Geometry: final body of the model. Coordinates: model frame, mm. A direction names the side the tool comes from. Round coordinates to 2 decimals unless told otherwise and drop trailing zeros. Write each loop counter-clockwise with the first axis right and the second up, starting at its lowest first coordinate (ties: lowest second). Pieces come first, ordered by that corner, then holes. Notation, with made-up numbers: M -22,66 L -13,66 A29 cw -13,90 Z; hole C 10.25,71 d4. An arc over 180 degrees is marked long. Put each result on its own line as item: value. Start each with the question number.
```python
from build123d import *

# Parameters (mm, degrees)
F0_W         = 127
F0_H         = 88.9
F1_DEPTH     = 50.8
F3_DEPTH     = 76.2
F4_W         = 76.2
F4_H         = 25.4
F5_DEPTH     = 38.1
F7_DEPTH     = 38.1
F8_T1_DEPTH  = 76.2
F8_T3_DEPTH  = 38.1
F8_T5_DEPTH  = 74.8723933942
F8_T8_ANGLE  = 242.9501193557
F8_T10_ANGLE = 242.9501193557
F8_T15_DEPTH = 38.1
F8_S16_R     = 24.2542650998
F8_T17_DEPTH = 21
F8_T21_DEPTH = 88.9
F8_S22_R     = 24.2542650998
F8_T23_DEPTH = 46
F8_T30_DEPTH = 88.9
F8_S32_R     = 29.6655396369
F8_T33_DEPTH = 46
F8_T36_DEPTH = 38.1
F8_S38_R     = 29.6655396369
F8_T39_DEPTH = 21


# Not quite as in the source:
# - a fillet or chamfer that OpenCascade refuses, or shapes differently, is made with other operations: its cross-section is extruded or revolved along the edge and cut away or added


with BuildPart() as f1:
    # F0 (on Top) → F1 (new body)
    with BuildSketch(Plane.XY):
        with Locations((0.947636019, -9.969078747)):
            Rectangle(F0_W, F0_H)
    extrude(amount=F1_DEPTH)

    # F2 (on face) → F3 (cut)
    with BuildSketch(Plane.XY.offset(50.8)):
        with BuildLine():
            Line((21.7591244727, 34.480921253), (-28.0215628445, 34.480921253))
            ThreePointArc((-28.0215628445, 34.480921253), (-3.1312191859, 8.6101276845), (21.7591244727, 34.480921253))
        make_face()
    extrude(amount=-F3_DEPTH, mode=Mode.SUBTRACT)

    # F4 (on face) → F5 (cut)
    with BuildSketch(Plane.XY.offset(50.8)):
        with Locations((0.8347104251, -41.719078747)):
            Rectangle(F4_W, F4_H)
    extrude(amount=-F5_DEPTH, mode=Mode.SUBTRACT)

    # F6 (on face) → F7 (cut)
    with BuildSketch(Plane.XY.offset(50.8)):
        with BuildLine():
            Line((-62.552363981, -54.419078747), (-49.9088267779, -54.419078747))
            Line((-49.9088267779, -54.419078747), (-49.9088267779, -29.019078747))
            ThreePointArc((-49.9088267779, -29.019078747), (-39.401677619, -18.2031822516), (-35.5692207813, -3.619078747))
            Line((-35.5692207813, -3.619078747), (-35.5692207813, 34.480921253))
            Line((-35.5692207813, 34.480921253), (-62.552363981, 34.480921253))
            Line((-62.552363981, 34.480921253), (-62.552363981, -54.419078747))
        make_face()
        with BuildLine():
            Line((51.6911732221, -27.8206840158), (51.6911732221, -54.419078747))
            Line((51.6911732221, -54.419078747), (64.447636019, -54.419078747))
            Line((64.447636019, -54.419078747), (64.447636019, 34.480921253))
            Line((64.447636019, 34.480921253), (29.0343053639, 34.480921253))
            Line((29.0343053639, 34.480921253), (29.0343053639, -3.619078747))
            ThreePointArc((29.0343053639, -3.619078747), (35.5824546884, -20.1950505038), (51.6911732221, -27.8206840158))
        make_face()
    extrude(amount=-F7_DEPTH, mode=Mode.SUBTRACT)

    # F8: fillet of radius 5.08 on 8 edges, made by hand

    # F8_s2 → F8_t1 (cut)
    with BuildSketch(Plane.YZ.offset(-37.2652895749)):
        with BuildLine():
            ThreePointArc((-23.939078747, 50.8), (-27.5311811954, 49.3121024484), (-29.019078747, 45.72))
            Line((-29.019078747, 45.72), (-29.019078747, 50.8))
            Line((-29.019078747, 50.8), (-23.939078747, 50.8))
        make_face()
        with BuildLine():
            ThreePointArc((-54.419078747, 7.62), (-52.9311811954, 11.2121024484), (-49.339078747, 12.7))
            Line((-49.339078747, 12.7), (-54.419078747, 12.7))
            Line((-54.419078747, 12.7), (-54.419078747, 7.62))
        make_face()
    extrude(amount=F8_T1_DEPTH, mode=Mode.SUBTRACT)

    # F8_s4 → F8_t3 (cut)
    with BuildSketch(Plane.XZ.offset(29.019078747)):
        with BuildLine():
            ThreePointArc((-42.3452895749, 50.8), (-38.7531871264, 49.3121024484), (-37.2652895749, 45.72))
            Line((-37.2652895749, 45.72), (-37.2652895749, 50.8))
            Line((-37.2652895749, 50.8), (-42.3452895749, 50.8))
        make_face()
        with BuildLine():
            ThreePointArc((44.0147104251, 50.8), (40.4226079767, 49.3121024484), (38.9347104251, 45.72))
            Line((38.9347104251, 45.72), (38.9347104251, 50.8))
            Line((38.9347104251, 50.8), (44.0147104251, 50.8))
        make_face()
    extrude(amount=F8_T3_DEPTH, mode=Mode.SUBTRACT)

    # F8_s6 → F8_t5 (cut)
    with BuildSketch(Plane.XY.offset(-12.0361966971)):
        with BuildLine():
            ThreePointArc((26.5736031516, 34.480921253), (23.2372411895, 33.2317291127), (21.5417284952, 30.0985152915))
            ThreePointArc((21.5417284952, 30.0985152915), (21.7471113974, 32.2849220687), (21.7591244727, 34.480921253))
            Line((21.7591244727, 34.480921253), (26.5736031516, 34.480921253))
        make_face()
        with BuildLine():
            ThreePointArc((-32.8360415234, 34.480921253), (-29.4996795612, 33.2317291127), (-27.804166867, 30.0985152915))
            ThreePointArc((-27.804166867, 30.0985152915), (-28.0095497691, 32.2849220687), (-28.0215628445, 34.480921253))
            Line((-28.0215628445, 34.480921253), (-32.8360415234, 34.480921253))
        make_face()
    extrude(amount=F8_T5_DEPTH, mode=Mode.SUBTRACT)

    # F8_s7 → F8_t8 (revolve, cut)
    with BuildSketch(Plane(origin=(14.0725928873, 22.9868383553, 0), x_dir=(0, 0, 1), z_dir=(0.5221273689, 0.8528675224, 0))):
        with BuildLine():
            ThreePointArc((45.72, -45.0806506369), (49.3121024484, -46.5685481884), (50.8, -50.1606506369))
            Line((50.8, -50.1606506369), (50.8, -45.0806506369))
            Line((50.8, -45.0806506369), (45.72, -45.0806506369))
        make_face()
    revolve(axis=Axis((-3.1312191859, 33.5190498615, 50.8), (0, 0, 1)), revolution_arc=F8_T8_ANGLE, mode=Mode.SUBTRACT)

    # F8_s9 → F8_t10 (revolve, cut)
    with BuildSketch(Plane(origin=(14.0725928873, 22.9868383553, 0), x_dir=(0, 0, 1), z_dir=(0.5221273689, 0.8528675224, 0))):
        with BuildLine():
            ThreePointArc((0, -50.1606506369), (1.4878975516, -46.5685481884), (5.08, -45.0806506369))
            Line((5.08, -45.0806506369), (0, -45.0806506369))
            Line((0, -45.0806506369), (0, -50.1606506369))
        make_face()
    revolve(axis=Axis((-3.1312191859, 33.5190498615, 0), (0, 0, 1)), revolution_arc=F8_T10_ANGLE, mode=Mode.SUBTRACT)


with BuildPart() as f8_tool13:
    # F8_s14 → F8_t15 (new body)
    with BuildSketch(Plane.XZ.offset(54.419078747)):
        with BuildLine():
            ThreePointArc((44.0147104251, 50.8), (40.4226079767, 49.3121024484), (38.9347104251, 45.72))
            Line((38.9347104251, 45.72), (38.9347104251, 50.8))
            Line((38.9347104251, 50.8), (44.0147104251, 50.8))
        make_face()
    extrude(amount=-F8_T15_DEPTH)

    # F8_s16 → F8_t17 (cut, symmetric)
    with BuildSketch(Plane.XY.offset(48.3)):
        with Locations((53.2885704637, -3.619078747)):
            Circle(F8_S16_R)
    extrude(amount=F8_T17_DEPTH, both=True, mode=Mode.SUBTRACT)

    split(bisect_by=Plane.XZ.offset(29.019078747), keep=Keep.BOTTOM)


with BuildPart() as f8_tool19:
    # F8_s20 → F8_t21 (new body)
    with BuildSketch(Plane.YZ.offset(51.6347104251)):
        with BuildLine():
            ThreePointArc((-23.939078747, 50.8), (-27.5311811954, 49.3121024484), (-29.019078747, 45.72))
            Line((-29.019078747, 45.72), (-29.019078747, 50.8))
            Line((-29.019078747, 50.8), (-23.939078747, 50.8))
        make_face()
    extrude(amount=-F8_T21_DEPTH)

    # F8_s22 → F8_t23 (cut, symmetric)
    with BuildSketch(Plane.XY.offset(48.3)):
        with Locations((53.2885704637, -3.619078747)):
            Circle(F8_S22_R)
    extrude(amount=F8_T23_DEPTH, both=True, mode=Mode.SUBTRACT)

    split(bisect_by=Plane.YZ.offset(38.9347104251), keep=Keep.TOP)


with BuildPart() as f8_tool13_1:
    add(f8_tool13.part)

    # F8_t25: intersect F8_tool19
    add(f8_tool19.part, mode=Mode.INTERSECT)


with BuildPart() as f1_1:
    add(f1.part)

    # F8_t11: cut F8_tool13
    add(f8_tool13_1.part, mode=Mode.SUBTRACT)


with BuildPart() as f8_tool28:
    # F8_s29 → F8_t30 (new body)
    with BuildSketch(Plane.YZ.offset(38.9347104251)):
        with BuildLine():
            ThreePointArc((-23.939078747, 50.8), (-27.5311811954, 49.3121024484), (-29.019078747, 45.72))
            Line((-29.019078747, 45.72), (-29.019078747, 50.8))
            Line((-29.019078747, 50.8), (-23.939078747, 50.8))
        make_face()
    extrude(amount=-F8_T30_DEPTH)

    split(bisect_by=Plane.YZ.offset(-37.2652895749), keep=Keep.BOTTOM)

    # F8_s32 → F8_t33 (cut, symmetric)
    with BuildSketch(Plane.XY.offset(48.3)):
        with Locations((-65.2347604182, -3.619078747)):
            Circle(F8_S32_R)
    extrude(amount=F8_T33_DEPTH, both=True, mode=Mode.SUBTRACT)


with BuildPart() as f8_tool34:
    # F8_s35 → F8_t36 (new body)
    with BuildSketch(Plane.XZ.offset(16.319078747)):
        with BuildLine():
            ThreePointArc((-42.3452895749, 50.8), (-38.7531871264, 49.3121024484), (-37.2652895749, 45.72))
            Line((-37.2652895749, 45.72), (-37.2652895749, 50.8))
            Line((-37.2652895749, 50.8), (-42.3452895749, 50.8))
        make_face()
    extrude(amount=F8_T36_DEPTH)

    split(bisect_by=Plane.XZ.offset(29.019078747), keep=Keep.BOTTOM)

    # F8_s38 → F8_t39 (cut, symmetric)
    with BuildSketch(Plane.XY.offset(48.3)):
        with Locations((-65.2347604182, -3.619078747)):
            Circle(F8_S38_R)
    extrude(amount=F8_T39_DEPTH, both=True, mode=Mode.SUBTRACT)


with BuildPart() as f8_tool28_1:
    add(f8_tool28.part)

    # F8_t40: intersect F8_tool34
    add(f8_tool34.part, mode=Mode.INTERSECT)


with BuildPart() as f1_2:
    add(f1_1.part)

    # F8_t26: cut F8_tool28
    add(f8_tool28_1.part, mode=Mode.SUBTRACT)


solid = f1_2.part
```
1) Section D-D, the plane y = -16. Output: boundary loops of the cut face in (x, z), and give its area (3 significant figures).
2) Access query for faces 4 (the face through (51.691, -41, 32)), 5 (the face through (35.4, -20, 32)), 6 (the face through (-52, 1, 12.7)), 7 (the face through (-29.538, 33.265, 25.044)), 8 (the face through (-49.909, -42, 32)). Directions: +Z, -Z, +X, -X, +Y, -Y. A direction counts if a zero-diameter tool reaches every point of the face in a straight line with its end or side. Return the directions, or none.
3) Ray query, probe 1 along Z at (x, y) = (-40, 25.5); probe 2 along X at (y, z) = (0, 14); probe 3 along X at (y, z) = (22.5, 46). Return the intervals inside material, ascending.
4) Section A-A, the plane y = -43. Output: boundary loops of the cut face in (x, z).
5) First-contact query: pin 1 (7.5 mm diameter, centred on y = -43.5, z = 23, fed in from -X); pin 2 (6 mm diameter, centred on x = -9, y = -45, fed in from +Z); pin 3 (6 mm diameter, centred on y = -34.5, z = 40.5, fed in from +X). Flat tips, straight axial feed; report the tip coordinate or a pass-through.
6) Section C-C, the plane y = -1. Output: boundary loops of the cut face in (x, z), and give its area (3 significant figures).
7) Section B-B, the plane z = 38.5. Output: boundary loops of the cut face in (x, y).
8) Draft query along X for faces 1 (the face through (40.46, -39.7, 49.35)), 2 (the face through (-35.569, 15, 32)), 3 (the face through (29.034, 16, 32)). Return one class per face: +X half, -X half, draft (parallel to the pull), parting line (faces both ways), or undercut.
Solved:
1. outline: M -62.55,0 L 64.45,0 L 64.45,12.7 L 32.43,12.7 L 32.43,50.8 L -38.28,50.8 L -38.28,12.7 L -62.55,12.7 Z
1. area: 4,310 mm2
2. face 4: +Z, +X, +Y, -Y
2. face 5: +Z, +X, +Y
2. face 6: +Z, -X, +Y
2. face 7: +Z, -Z, +Y
2. face 8: +Z, -X, +Y, -Y
3. probe 1: z = 0 to 12.7
3. probe 2: x = -35.57 to 29.03
3. probe 3: x = -35.57 to -25.48, 19.22 to 29.03
4. outline: M -62.55,0 L 64.45,0 L 64.45,12.7 L 51.69,12.7 L 51.69,50.8 L 44.01,50.8 A5.08 ccw 38.93,45.72 L 38.93,12.7 L -37.27,12.7 L -37.27,45.72 A5.08 ccw -42.35,50.8 L -49.91,50.8 L -49.91,12.7 L -62.55,12.7 Z
5. pin 1: stops at x = -49.91
5. pin 2: stops at z = 12.7
5. pin 3: stops at x = 51.69
6. outline: M -62.55,0 L 64.45,0 L 64.45,12.7 L 29.03,12.7 L 29.03,50.8 L -35.57,50.8 L -35.57,12.7 L -62.55,12.7 Z
6. area: 4,070 mm2
7. outline: M -49.91,-54.42 L -37.27,-54.42 L -37.27,-29.02 L 38.93,-29.02 L 38.93,-54.42 L 51.69,-54.42 L 51.69,-27.82 A24.25 cw 29.03,-3.62 L 29.03,34.48 L 26.57,34.48 A5.08 ccw 21.54,30.1 A24.91 cw -27.8,30.1 A5.08 ccw -32.84,34.48 L -35.57,34.48 L -35.57,-3.62 A29.67 cw -49.91,-29.02 Z
8. face 1: undercut
8. face 2: -X half
8. face 3: +X half
